Autodesk Inventor part; units mm, degrees
ref_plane "YZ Plane" through (0, 0, 0) normal (1, 0, 0) x (0, 1, 0)
ref_plane "XZ Plane" through (0, 0, 0) normal (0, 1, 0) x (-1, 0, 0)
ref_plane "XY Plane" through (0, 0, 0) normal (0, 0, 1) x (1, 0, 0)
sketch "Sketch2" plane through (0, 0, 0) normal (0, 1, 0) x (-1, 0, 0)
  line L0 (-51.5, -51.5) -> (51.5, -51.5)
  line L1 (51.5, -51.5) -> (51.5, 51.5)
  line L2 (51.5, 51.5) -> (-51.5, 51.5)
  line L3 (-51.5, 51.5) -> (-51.5, -51.5)
  line L4 (-51.5, -51.5) -> (51.5, 51.5) construction
  line L5 (51.5, -51.5) -> (-51.5, 51.5) construction
  point P0 (0, 0)
  dimension "d6" = 103
  dimension "d7" = 103
extrude "Extrusion2" add sketch "Sketch2" along normal blind 9
fillet "Fillet3" radius 30 1 edges at (-51.5, 4.5, -51.5)
fillet "Fillet4" radius 30 1 edges at (51.5, 4.5, -51.5)
fillet "Fillet5" radius 30 1 edges at (-51.5, 4.5, 51.5)
sketch "Sketch3" plane through (0, 0, 0) normal (0, -1, 0) x (1, 0, 0)
  line L0 (51.5, 51.5) -> (51.5, -21.5)
  line L1 (21.5, -51.5) -> (-21.5, -51.5)
  line L2 (51.5, 51.5) -> (18.5, 51.5)
  line L3 (18.5, 51.5) -> (18.5, -51.5)
  line L4 (18.5, -51.5) -> (51.5, -51.5)
  line L5 (51.5, -51.5) -> (51.5, 51.5)
  point P0 (0, 0)
  dimension "d13" = 33
extrude "Extrusion3" cut sketch "Sketch3" against normal blind 9
sketch "Sketch4" plane through (0, 0, 0) normal (0, -1, 0) x (1, 0, 0)
  line L0 (-21.5, 51.5) -> (18.5, 51.5)
  line L1 (18.5, 51.5) -> (18.5, 25.5)
  line L2 (18.5, 51.5) -> (18.5, -51.5)
  line L3 (18.5, -51.5) -> (18.5, -25.5)
  line L4 (18.5, 25.5) -> (4.5, 25.5)
  line L5 (4.5, 25.5) -> (4.5, -25.5)
  line L6 (4.5, -25.5) -> (18.5, -25.5)
  line L7 (18.5, -25.5) -> (18.5, 25.5)
  point P0 (0, 0)
  dimension "d16" = 26
  dimension "d17" = 26
  dimension "d18" = 14
extrude "Extrusion4" cut sketch "Sketch4" against normal blind 9
sketch "Sketch5" plane through (0, 0, 0) normal (0, -1, 0) x (1, 0, 0)
  line L0 (18.5, 51.5) -> (18.5, 33.5)
  line L1 (18.5, 25.5) -> (18.5, 51.5)
  line L2 (4.5, 25.5) -> (4.5, -25.5)
  line L3 (18.5, 33.5) -> (4.5, 25.5)
  line L4 (18.5, 25.5) -> (4.5, 25.5)
  line L5 (4.5, 25.5) -> (18.5, 25.5)
  line L6 (18.5, 25.5) -> (18.5, 33.5)
  line L7 (18.5, -51.5) -> (-21.5, -51.5)
  line L8 (18.5, -51.5) -> (18.5, -33.5)
  line L9 (18.5, -25.5) -> (18.5, -51.5)
  line L10 (18.5, -33.5) -> (4.5, -25.5)
  line L11 (4.5, -25.5) -> (18.5, -25.5)
  line L12 (18.5, -25.5) -> (18.5, -33.5)
  point P0 (0, 0)
  dimension "d21" = 18
  dimension "d22" = 18
extrude "Extrusion5" cut sketch "Sketch5" against normal blind 9
fillet "Fillet6" radius 4 4 edges at (4.5, 4.5, 25.5) (18.5, 4.5, 33.5) (18.5, 4.5, -33.5) (4.5, 4.5, -25.5)
sketch "Sketch6" plane through (0, 0, 0) normal (0, -1, 0) x (1, 0, 0)
  line L0 (-21.5, 51.5) -> (18.5, 51.5)
  line L1 (18.5, 51.5) -> (18.5, 43)
  line L2 (18.5, 35.8213) -> (18.5, 51.5)
  line L3 (18.5, 43) -> (15, 43)
  circle A0 centre (15, 43) radius 2.5
  line L4 (18.5, -51.5) -> (-21.5, -51.5)
  line L5 (18.5, -51.5) -> (18.5, -43)
  line L6 (18.5, -35.8213) -> (18.5, -51.5)
  line L7 (18.5, -43) -> (15, -43)
  circle A1 centre (15, -43) radius 2.5
  line L8 (18.5, -51.5) -> (-5.5, -51.5)
  line L9 (-5.5, -51.5) -> (-5.5, -46)
  circle A2 centre (-5.5, -46) radius 2.5
  line L10 (18.5, 51.5) -> (-5.5, 51.5)
  line L11 (-5.5, 51.5) -> (-5.5, 46)
  circle A3 centre (-5.5, 46) radius 2.5
  point P0 (0, 0)
  dimension "d26" = 8.5
  dimension "d27" = 3.5
  dimension "d28" = 5
  dimension "d29" = 8.5
  dimension "d30" = 5
  dimension "d31" = 24
  dimension "d32" = 5.5
  dimension "d33" = 5
  dimension "d34" = 5.5
extrude "Extrusion6" cut sketch "Sketch6" against normal blind 9
sketch "Sketch7" plane through (0, 0, 0) normal (0, -1, 0) x (1, 0, 0)
  line L0 (4.5, 23.1787) -> (4.5, -23.1787)
  line L1 (4.5, 0) -> (-5.5, 0)
  circle A0 centre (-5.5, 0) radius 5
  circle A1 centre (-5.5, 0) radius 17
  point P0 (0, 0)
  dimension "d37" = 10
  dimension "d38" = 34
extrude "Extrusion7" cut sketch "Sketch7" against normal blind 4
sketch "Sketch8" plane through (-5.5, 0, 0) normal (0, -1, 0) x (1, 0, 0)
  circle A0 centre (0, 0) radius 5
  point P0 (5.5, 0)
extrude "Extrusion8" cut sketch "Sketch8" against normal blind 5
sketch "Sketch9" plane through (0, 0, 0) normal (0, -1, 0) x (1, 0, 0)
  line L0 (-21.5, 51.5) -> (18.5, 51.5)
  arc A0 (-21.5, 51.5) -> (-51.5, 21.5) centre (-21.5, 21.5) ccw
  line L1 (-51.5, -21.5) -> (-51.5, 21.5)
  arc A1 (-51.5, -21.5) -> (-21.5, -51.5) centre (-21.5, -21.5) ccw
  line L2 (18.5, -51.5) -> (-21.5, -51.5)
  line L3 (18.5, -46.5) -> (-21.5, -46.5)
  arc A2 (-46.5, -21.5) -> (-21.5, -46.5) centre (-21.5, -21.5) ccw
  line L4 (-46.5, -21.5) -> (-46.5, 21.5)
  arc A3 (-21.5, 46.5) -> (-46.5, 21.5) centre (-21.5, 21.5) ccw
  line L5 (-21.5, 46.5) -> (18.5, 46.5)
  arc A4 (4.5, 13.7477) -> (4.5, -13.7477) centre (-5.5, 0) ccw
  arc A5 (7.4412, 17.7912) -> (7.4412, -17.7912) centre (-5.5, 0) ccw
  arc A6 (-18.6225, 17.6579) -> (-25.2059, 46.2238) centre (-28.1661, 30.5) ccw
  arc A7 (-25.2059, -46.2238) -> (-18.6225, -17.6579) centre (-28.1661, -30.5) ccw
  arc A8 (5.9706, 15.7695) -> (5.9706, -15.7695) centre (-5.5, 0) ccw
  circle A9 centre (-5.5, 0) radius 5
  line L6 (-5.5, 0) -> (-21.5, 11.1467)
  line L7 (-5.5, 0) -> (-21.5, -11.1467)
  circle A10 centre (-21.5, 11.1467) radius 2.5
  circle A11 centre (-21.5, -11.1467) radius 2.5
  point P0 (0, 0)
  dimension "d43" = 5
  dimension "d44" = 5
  dimension "d45" = 32
  dimension "d46" = 32
  dimension "d47" = 2.5
extrude "Extrusion9" cut sketch "Sketch9" against normal blind 4 contours L4 A3 A6 A5 A7 A2
sketch "Sketch10" plane through (0, 0, 0) normal (0, -1, 0) x (1, 0, 0)
  arc A0 (4.5, 13.7477) -> (4.5, -13.7477) centre (-5.5, 0) ccw
  line L0 (-5.5, 0) -> (-21.1252, 11.6663)
  line L1 (-5.5, 0) -> (-21.1252, -11.6663)
  line L2 (-21.1252, 11.6663) -> (-23.1284, 13.162)
  arc A1 (-18.6225, 17.6579) -> (-18.6225, -17.6579) centre (-5.5, 0) ccw
  line L3 (-21.1252, -11.6663) -> (-23.1284, -13.162)
  arc A2 (-19.122, 10.1707) -> (-19.122, -10.1707) centre (-5.5, 0) ccw
  arc A3 (7.4412, 17.7912) -> (7.4412, -17.7912) centre (-5.5, 0) ccw
  arc A4 (-19.122, 10.1707) -> (-19.122, -10.1707) centre (-5.5, 0) ccw
  point P0 (0, 0)
  dimension "d52" = 5
  dimension "d53" = 5
extrude "Extrusion10" cut sketch "Sketch10" against normal blind 4 contours A0 L1 L3 A1 L2 L0
sketch "Sketch11" plane through (0, 4, 0) normal (0, -1, 0) x (1, 0, 0)
  line L0 (-23.1284, 13.162) -> (-19.122, 10.1707)
  circle A0 centre (-21.1252, 11.6663) radius 2.5
  line L1 (-19.122, -10.1707) -> (-23.1284, -13.162)
  circle A1 centre (-21.1252, -11.6663) radius 2.5
  point P0 (0, 0)
  dimension "d56" = 5
  dimension "d57" = 5
extrude "Extrusion11" add sketch "Sketch11" along normal blind 4
fillet "Fillet7" radius 14 1 edges at (-25.2059, 2, -46.2238)
fillet "Fillet8" radius 14 1 edges at (-25.2059, 2, 46.2238)
sketch "Sketch12" plane through (0, 4, 0) normal (0, -1, 0) x (1, 0, 0)
  line L0 (-46.5, -21.5) -> (-46.5, 21.5)
  line L1 (-46.5, 0) -> (-31.5, 0)
  line L2 (-31.5, 0) -> (-31.5, 10)
  line L3 (-31.5, 10) -> (-46.5, 10)
  line L4 (-46.5, 10) -> (-46.5, 0)
  line L5 (-46.5, 0) -> (-31.5, 0)
  line L6 (-31.5, 0) -> (-31.5, -10)
  line L7 (-31.5, -10) -> (-46.5, -10)
  line L8 (-46.5, -10) -> (-46.5, 0)
  arc A0 (-36.4424, -5.9061) -> (-36.1425, 5.8444) centre (-37.5, 0) ccw
  line L9 (-46.5, 10) -> (-46.5, -10)
  line L10 (-46.5, -10) -> (-36.4424, -5.9061)
  line L11 (-46.5, 10) -> (-36.1425, 5.8444)
  line L12 (-46.5, 10) -> (-46.5, -10)
  point P0 (0, 0)
  dimension "d62" = 15
  dimension "d63" = 10
  dimension "d64" = 15
  dimension "d65" = 10
  dimension "d66" = 12
extrude "Extrusion12" add sketch "Sketch12" along normal blind 4 contours L0 L1 A0 L10 | L0 L11 A0 L1
fillet "Fillet9" radius 4 2 edges at (-46.5, 2, -10) (-46.5, 2, 10)
sketch "Sketch13" plane through (0, 0, 0) normal (0, -1, 0) x (1, 0, 0)
  arc A0 (-36.4424, -5.9061) -> (-36.1425, 5.8444) centre (-37.5, 0) ccw
  arc A1 (-37.1475, -1.9687) -> (-37.0475, 1.9481) centre (-37.5, 0) ccw
  circle A2 centre (-37.5, 0) radius 2
  line L0 (-51.5, -21.5) -> (-51.5, 21.5)
  line L1 (-51.5, 0) -> (-46.5, 0)
  line L2 (-46.5, 3.5) -> (-46.5, 6)
  line L3 (-46.5, -3.5) -> (-46.5, -6)
  arc A3 (-44, 6) -> (-49, 6) centre (-46.5, 6) ccw
  arc A4 (-49, -6) -> (-44, -6) centre (-46.5, -6) ccw
  line L4 (-44, -6) -> (-44, 6)
  line L5 (-49, 6) -> (-49, -6)
  point P0 (0, 0)
  dimension "d70" = 4
  dimension "d71" = 5
  dimension "d72" = 6
  dimension "d73" = 6
  dimension "d74" = 5
  dimension "d75" = 5
extrude "Extrusion13" cut sketch "Sketch13" against normal blind 9
properties part number "Kompliteringsbit"
The model under review builds one solid part; all positions refer to its coordinate system, in mm. A direction names the side the tool comes from. Coordinates: 2 decimals unless noted, no trailing zeros. Order: outer loops, then holes, each group sorted by start corner. A loop starts at its lowest first (then second) coordinate and runs counter-clockwise, first axis right, second up. Notation, with made-up numbers: (74.5, 31) -> (115.5, 31) arc R16 ccw to (115.5, 59) -> close; hole circle Ø1 at (2.25, 88.5). An arc over 180 degrees is marked (long way). Answer in a Markdown table with one row per item.
(1) Consider section B-B (z = 0). Write out the cut boundary in (x, y).
Answers:
| item | result |
|---|---|
| outline | (-51.5, 0) -> (-49, 0) -> (-49, 9) -> (-51.5, 9) -> close; (-44, 0) -> (-39.5, 0) -> (-39.5, 9) -> (-44, 9) -> close; (-35.5, 0) -> (-31.5, 0) -> (-31.5, 4) -> (-10.5, 4) -> (-10.5, 5) -> (-0.5, 5) -> (-0.5, 4) -> (4.5, 4) -> (4.5, 9) -> (-35.5, 9) -> close |
(2) Wall thickness on line 1 along X through (y, z) = (3.5, 0); line 2 along X through (y, z) = (6, 0); line 3 along Z through (x, y) = (15, 7): over which ranges is each line inside the solid? List them lowest first.
Answers:
| item | result |
|---|---|
| line 1 | -51.5 to -49, -44 to -39.5, -35.5 to -31.5 |
| line 2 | -51.5 to -49, -44 to -39.5, -35.5 to 4.5 |
| line 3 | -51.5 to -45.5, -40.5 to -31.5, 31.5 to 40.5, 45.5 to 51.5 |
(3) Consider section D-D (y = 6). Write out the cut boundary in (x, z), plus the area to 3 significant figures.
Answers:
| item | result |
|---|---|
| outline | (-51.5, -21.5) arc R30 ccw to (-21.5, -51.5) -> (18.5, -51.5) -> (18.5, -35.82) arc R4 ccw to (16.48, -32.35) -> (6.52, -26.65) arc R4 cw to (4.5, -23.18) -> (4.5, 23.18) arc R4 cw to (6.52, 26.65) -> (16.48, 32.35) arc R4 ccw to (18.5, 35.82) -> (18.5, 51.5) -> (-21.5, 51.5) arc R30 ccw to (-51.5, 21.5) -> close; hole (-49, -6) arc R2.5 ccw to (-44, -6) -> (-44, 6) arc R2.5 ccw to (-49, 6) -> close; hole (-37.15, -1.97) arc R2 ccw to (-37.05, 1.95) arc R2 ccw (long way) to start; hole circle Ø5 at (-5.5, -46); hole circle Ø5 at (-5.5, 46); hole circle Ø5 at (15, -43); hole circle Ø5 at (15, 43) |
| area | 5,830 mm² |
(4) Consider section C-C (x = -5.5). Write out the cut boundary in (y, z).
Answers:
| item | result |
|---|---|
| outline | (0, -51.5) -> (9, -51.5) -> (9, -48.5) -> (0, -48.5) -> close; (0, -43.5) -> (9, -43.5) -> (9, 43.5) -> (0, 43.5) -> (0, 17) -> (4, 17) -> (4, 5) -> (5, 5) -> (5, -5) -> (4, -5) -> (4, -17) -> (0, -17) -> close; (0, 48.5) -> (9, 48.5) -> (9, 51.5) -> (0, 51.5) -> close |
(5) Consider section A-A (x = 8). Write out the cut boundary in (y, z).
Answers:
| item | result |
|---|---|
| outline | (0, -51.5) -> (9, -51.5) -> (9, -27.5) -> (0, -27.5) -> close; (0, 27.5) -> (9, 27.5) -> (9, 51.5) -> (0, 51.5) -> close |
(6) Machinability: for faces 4 (the flat face through (-40.12, 2.03, 7.44)), 5 (the cylindrical face through (-21.007, 1.972, 15.605)), 6 (the cylindrical face through (-46.6, 4.4, -8.5)), which of the approach directions +Z, -Z, +X, -X, +Y, -Y give a long, thin tool a straight path to every point of the face, cutting with its end or side? Answer none if there is none.
Answers:
| item | result |
|---|---|
| face 4 | +X, -Y |
| face 5 | -Y |
| face 6 | +Y, -Y |
(7) The part is to be moulded in two halves that separate along Z. For faces 1 (the flat face through (-27, 4, 1)), 2 (the cylindrical face through (-42.479, 4.563, -42.945)), 3 (the flat face through (-32, 0, 1)), say which applies: +Z half, -Z half, draft (parallel to the pull), parting line (faces both ways), or undercut.
Answers:
| item | result |
|---|---|
| face 1 | undercut |
| face 2 | -Z half |
| face 3 | draft |
(8) Insertion check: pin 1 (4.5 mm diameter, centred on x = -5.5, z = 46, fed in from -Y); pin 2 (12 mm diameter, centred on x = 5.5, z = -6.5, fed in from +Y); pin 3 (4 mm diameter, centred on x = -26, y = 3.5, fed in from +Z); pin 4 (1.2 mm diameter, centred on y = 2.5, z = 15, fed in from +X). Each pin has a flat end and moves straight along its axis. Give the tip position at first contact, or say it passes through.
Answers:
| item | result |
|---|---|
| pin 1 | through |
| pin 2 | y = 9 |
| pin 3 | z = 51.4 |
| pin 4 | x = 4.5 |
